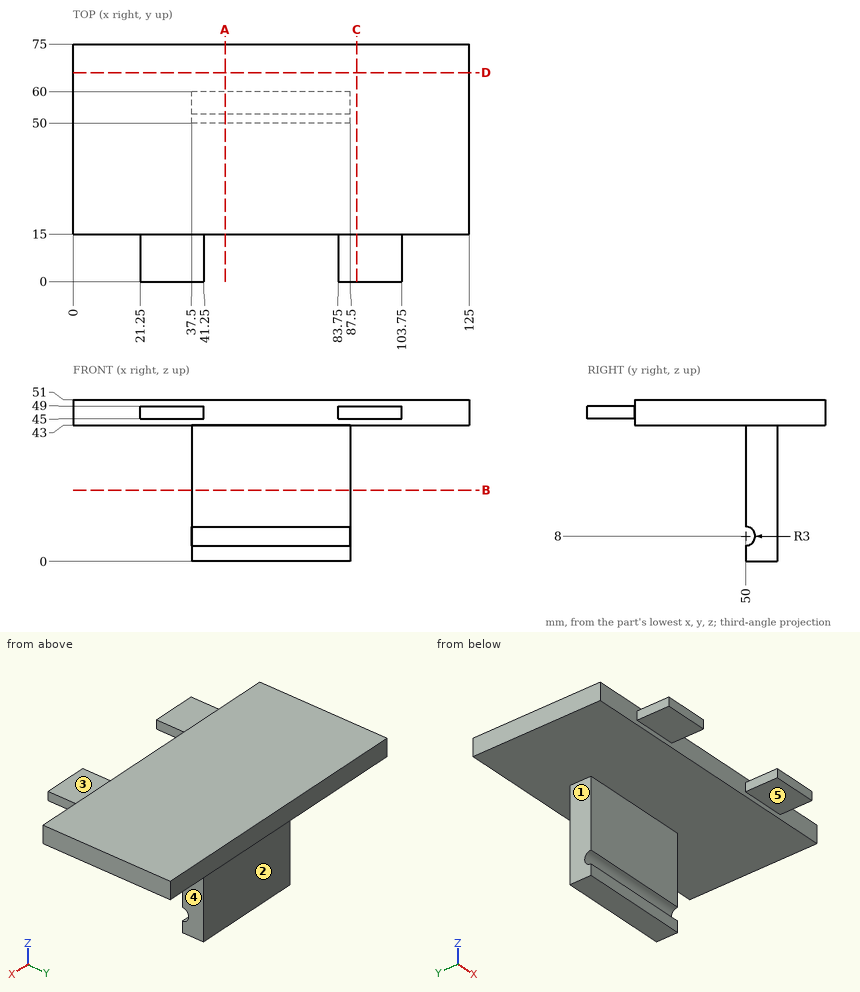
Part print with two shaded views. Sizes in mm from the minimum x, y, z corner. A direction names the side the tool comes from. Round coordinates to 2 decimals unless told otherwise and drop trailing zeros. Loops run counter-clockwise (first coordinate to the right, second up) from the corner with the lowest first, then second, coordinate; pieces in that order, holes last. Notation, with made-up numbers: M 65.25,13.5 L 94.25,13.5 A19 ccw 94.25,23.5 Z; hole C -16,-17.75 d8. An arc over 180 degrees is marked long. Return JSON: item names as keys, results as strings. Group by question number.
(1) Drop flat-ended pins along their axis: P1, Ø1.5, axis at x = 55.5, z = 3, coming from the -Y side; P2, Ø5, axis at y = 56, z = 15.5, coming from the +X side; P3, Ø3, axis at y = 7, z = 47, coming from the +X side. Give the stop position or say it passes through.
(2) Saw through at B-B, the plane z = 22.5. List the corners of the cut face in (x, y), and give its area (3 significant figures).
(3) Wall check: probe 1 along X at (y, z) = (56.5, 28); probe 2 along Z at (x, y) = (45.5, 41); probe 3 along Y at (x, z) = (107, 47). Give the ranges that are in metal, low to high. Write a range as [from, to].
(4) Saw through at C-C, the plane x = 89.5. List the corners of the cut face in (y, z).
(5) Tool access for the marked faces 1, 2, 3, 4 and 5: list every direction of +Z, -Z, +X, -X, +Y, -Y with a clear straight run to the whole face (end or side of a thin tool).
(6) Saw through at A-A, the plane x = 48. List the corners of the cut face in (y, z).
(7) Saw through at D-D, the plane y = 66. List the corners of the cut face in (x, z), and give its area (3 significant figures).
Answer list:
{
 "1": {"P1": "y = 50", "P2": "x = 87.5", "P3": "x = 103.75"},
 "2": {"outline": "M 37.5,50 L 87.5,50 L 87.5,60 L 37.5,60 Z", "area": "500 mm2"},
 "3": {"probe 1": "[37.5, 87.5]", "probe 2": "[43, 51]", "probe 3": "[15, 75]"},
 "4": {"outline": "M 0,45 L 15,45 L 15,43 L 75,43 L 75,51 L 15,51 L 15,49 L 0,49 Z"},
 "5": {"face 1": "-Z, -X, +Y, -Y", "face 2": "-Z, +X, -X, +Y", "face 3": "+Z, +X, -X, -Y", "face 4": "-Z, +X, +Y, -Y", "face 5": "-Z, +X, -X, -Y"},
 "6": {"outline": "M 15,43 L 50,43 L 50,11 A3 cw 50,5 L 50,0 L 60,0 L 60,43 L 75,43 L 75,51 L 15,51 Z"},
 "7": {"outline": "M 0,43 L 125,43 L 125,51 L 0,51 Z", "area": "1,000 mm2"}
}
